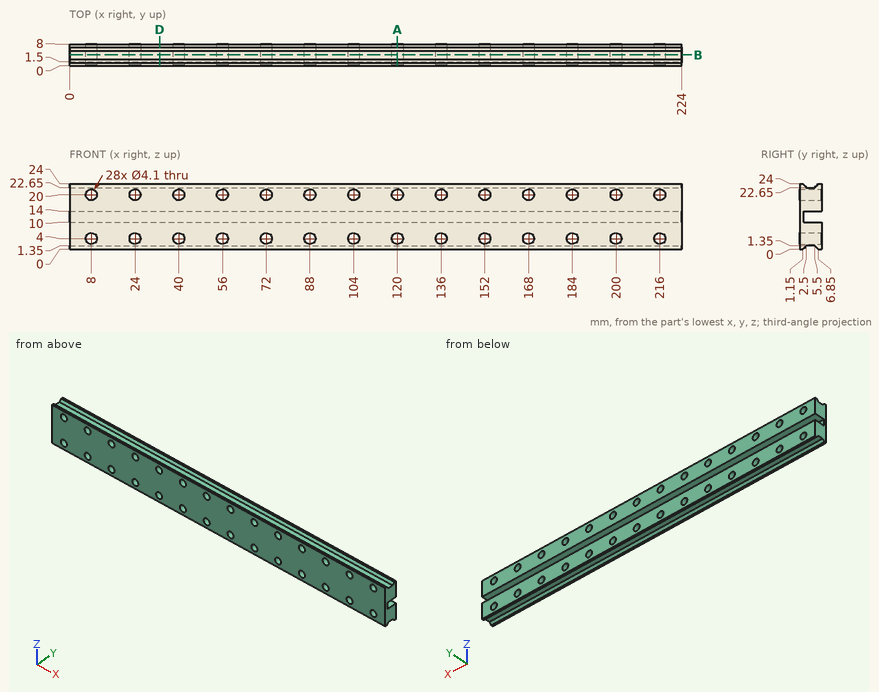
Part print with two shaded views. Sizes in mm from the minimum x, y, z corner. Round coordinates to 2 decimals unless told otherwise and drop trailing zeros. Write each loop counter-clockwise with the first axis right and the second up, starting at its lowest first coordinate (ties: lowest second). Pieces come first, ordered by that corner, then holes. Notation, with made-up numbers: (32, 25.5) -> (55, 25.5) arc R12 cw to (55, 44.5) -> close; hole circle Ø6 at (-27.5, -4.75). An arc over 180 degrees is marked (long way). Use one line per item in the form item = value.
Q1. Drill centre lines: L1, parallel to Z at x = 118.5, y = 0.75; L2, parallel to Z at x = 72, y = 6; L3, parallel to Y at x = 141.5, z = 13.75. Where is each one in solid material? Low to high.
Conclusion:
L1 = 0 to 2.6, 5.4 to 18.6, 21.4 to 24
L2 = 0.85 to 1.95, 6.05 to 10, 14 to 17.95, 22.05 to 23.15
L3 = 0 to 1.5
Q2. Band-saw the part on B-B, the plane y = 4. State how many separate pieces and enclosed holes the cut face has, then the cut area to 3 significant figures.
Conclusion:
separate_pieces = 2
enclosed_holes = 28
area = 3,510 mm²
Q3. Band-saw the part on D-D, the plane x = 33. Write the cut outline in (y, z).
Conclusion:
outline = (0, 0) -> (1.15, 0) -> (2.5, 1.35) -> (5.5, 1.35) -> (6.85, 0) -> (8, 0) -> (8, 10) -> (1.5, 10) -> (1.5, 14) -> (8, 14) -> (8, 24) -> (6.85, 24) -> (5.5, 22.65) -> (2.5, 22.65) -> (1.15, 24) -> (0, 24) -> close
Q4. Band-saw the part on A-A, the plane x = 120. Write the cut outline in (y, z).
Conclusion:
outline = (0, 0) -> (1.15, 0) -> (2.5, 1.35) -> (5.5, 1.35) -> (6.85, 0) -> (8, 0) -> (8, 1.95) -> (0, 1.95) -> close; (0, 6.05) -> (8, 6.05) -> (8, 10) -> (1.5, 10) -> (1.5, 14) -> (8, 14) -> (8, 17.95) -> (0, 17.95) -> close; (0, 22.05) -> (8, 22.05) -> (8, 24) -> (6.85, 24) -> (5.5, 22.65) -> (2.5, 22.65) -> (1.15, 24) -> (0, 24) -> close
Q5. Drop flat-ended pins along their axis: P1, Ø2.5, axis at x = 142.5, y = 3.5, coming from the +Z side; P2, Ø1.5, axis at x = 106.5, y = 4.5, coming from the -Z side. Give the stop position or say it passes through.
Conclusion:
P1 = 22.9
P2 = 1.35
